```python
from build123d import *

# Parameters (mm, degrees)
SKETCH1_W            = 157.0786
SKETCH1_H            = 90.551
BOSS_EXTRUDE1_DEPTH  = 8
CUT_EXTRUDE21_DEPTH  = 5
FILLET8_R            = 2.75
SKETCH29_W           = 11.58993
SKETCH29_H           = 90.551
CUT_EXTRUDE25_DEPTH  = 182.486005463
FILLET9_R            = 5
SKETCH36_W           = 10
SKETCH36_H           = 10
SKETCH36_R           = 3.3
BOSS_EXTRUDE10_DEPTH = 8
FILLET10_R           = 2.5
CUT_EXTRUDE26_DEPTH  = 3


with BuildPart() as part:
    # Sketch1 → Boss-Extrude1 (new body)
    with BuildSketch(Plane(origin=(0, 0, 0), x_dir=(1, 0, 0), z_dir=(0, 1, 0))):
        with Locations((78.5393, -45.2755)):
            Rectangle(SKETCH1_W, SKETCH1_H)
    extrude(amount=BOSS_EXTRUDE1_DEPTH)

    # Sketch23 → Cut-Extrude21 (cut)
    with BuildSketch(Plane(origin=(0, 8, 0), x_dir=(1, 0, 0), z_dir=(0, 1, 0))):
        Polygon((140.6288, -86.4755), (23.2359173, -86.4755), (16.4498, -79.6893827), (16.4498, -10.8616173), (23.2359173, -4.0755), (140.6288, -4.0755), align=None)
    extrude(amount=-CUT_EXTRUDE21_DEPTH, mode=Mode.SUBTRACT)

    # Fillet8
    fillet8_edges = [part.edges().sort_by_distance(p)[0] for p in [
        (140.6288, 5.5, 4.0755),
        (140.6288, 5.5, 86.4755),
        (23.2359173, 5.5, 86.4755),
        (16.4498, 5.5, 79.6893827),
        (16.4498, 5.5, 10.8616173),
        (23.2359173, 5.5, 4.0755),
    ]]
    fillet(fillet8_edges, radius=FILLET8_R)

    # Sketch29 → Cut-Extrude25 (cut, through all)
    with BuildSketch(Plane(origin=(0, 8, 0), x_dir=(1, 0, 0), z_dir=(0, 1, 0))):
        with Locations((151.283635, -45.2755)):
            Rectangle(SKETCH29_W, SKETCH29_H)
        with Locations((5.794965, -45.2755)):
            Rectangle(SKETCH29_W, SKETCH29_H)
    extrude(amount=-CUT_EXTRUDE25_DEPTH, mode=Mode.SUBTRACT)

    # Fillet9
    fillet9_edges = [part.edges().sort_by_distance(p)[0] for p in [
        (145.48867, 4, 90.551),
        (145.48867, 4, 0),
        (11.58993, 4, 0),
        (11.58993, 4, 90.551),
    ]]
    fillet(fillet9_edges, radius=FILLET9_R)

    # Sketch36 → Boss-Extrude10 (add)
    # profile 1 of 4: a face of its own
    with BuildSketch(Plane.XZ):
        with Locations((25.6082, 95.551)):
            Rectangle(SKETCH36_W, SKETCH36_H)
        with Locations(Location((25.6082, 95.551, 0), (0, 0, 270))):
            Circle(SKETCH36_R, mode=Mode.SUBTRACT)
    # profile 2 of 4: a face of its own
    with BuildSketch(Plane.XZ):
        with Locations((128.3942697, 95.551)):
            Rectangle(SKETCH36_W, SKETCH36_H)
        with Locations(Location((128.3942697, 95.551, 0), (0, 0, 270))):
            Circle(SKETCH36_R, mode=Mode.SUBTRACT)
    # profile 3 of 4: a face of its own
    with BuildSketch(Plane.XZ):
        with Locations((25.6082, -5)):
            Rectangle(SKETCH36_W, SKETCH36_H)
        with Locations(Location((25.6082, -5, 0), (0, 0, 270))):
            Circle(SKETCH36_R, mode=Mode.SUBTRACT)
    # profile 4 of 4: a face of its own
    with BuildSketch(Plane.XZ):
        with Locations((128.3942697, -5)):
            Rectangle(SKETCH36_W, SKETCH36_H)
        with Locations(Location((128.3942697, -5, 0), (0, 0, 270))):
            Circle(SKETCH36_R, mode=Mode.SUBTRACT)
    extrude(amount=-BOSS_EXTRUDE10_DEPTH)

    # Fillet10
    fillet10_edges = [part.edges().sort_by_distance(p)[0] for p in [
        (20.6082, 4, 90.551),
        (20.6082, 4, 100.551),
        (30.6082, 4, 100.551),
        (30.6082, 4, 90.551),
        (123.3942697, 4, 90.551),
        (123.3942697, 4, 100.551),
        (133.3942697, 4, 100.551),
        (133.3942697, 4, 90.551),
        (30.6082, 4, 0),
        (30.6082, 4, -10),
        (20.6082, 4, -10),
        (20.6082, 4, 0),
        (123.3942697, 4, -10),
        (123.3942697, 4, 0),
        (133.3942697, 4, 0),
        (133.3942697, 4, -10),
    ]]
    fillet(fillet10_edges, radius=FILLET10_R)

    # Sketch37 → Cut-Extrude26 (cut)
    with BuildSketch(Plane(origin=(0, 3, 0), x_dir=(1, 0, 0), z_dir=(0, 1, 0))):
        Polygon((21.1393, -77.618314888), (24.996485112, -81.4755), (135.9393, -81.4755), (135.9393, -9.0755), (24.996485112, -9.0755), (21.1393, -12.932685112), align=None)
    extrude(amount=-CUT_EXTRUDE26_DEPTH, mode=Mode.SUBTRACT)


solid = part.part
```
Geometry check sheet. Reference: the model listing, model coordinates, mm. A direction names the side the tool comes from. Give positions to 0.01 mm unless a question says otherwise; leave off trailing zeros. Order: outer loops, then holes, each group sorted by start corner. A loop starts at its lowest first (then second) coordinate and runs counter-clockwise, first axis right, second up.
1. Gauge pin test, flat ends, axial feed: pin 1 Ø2 at (x, y) = (36, 6.5) entering from +Z; pin 2 Ø7.5 at (x, z) = (128.39, -5) entering from -Y; pin 3 Ø1.5 at (y, z) = (2, 95.5) entering from +X; pin 4 Ø1.5 at (x, y) = (124.5, 2.5) entering from +Z. Record the tip position at first contact, or that the pin passes through.
2. Access from +Z, -Z, +X, -X, +Y, -Y to the whole of each face (thin tool, end or side, straight path). Record for faces 4 (the face through (133.394, 4, 96)), 5 (the face through (123.394, 4, 96)), 6 (the face through (133.394, 4, -5)), 7 (the face through (20.608, 4, 96)).
3. Section check B-B, the plane z = -5. Enter the section's corners in (x, y), and give its area (3 significant figures).
4. Thickness scan on L1, parallel to X at y = 1.5, z = -5; L2, parallel to Z at x = 88.5, y = 4; L3, parallel to Z at x = 117.5, y = 1.75. Record the ranges inside material, lowest first.
5. Release check for a two-part mould opening along Z. For faces 1 (the face through (79, 3, 82)), 2 (the face through (30.608, 4, -5)), 3 (the face through (76, 4, 0)) record: pulls with the +Z half, pulls with the -Z half, needs draft (parallel to the pull), parting line crosses it, or undercut.
6. Section check A-A, the plane x = 73. Enter the section's corners in (y, z).
7. Section check D-D, the plane y = 1.5. Give the number of separate pieces and of enclosed holes in the cut face, and give its area (3 significant figures).
8. Section check C-C, the plane z = 15. Enter the section's corners in (x, y).
Values follow:
1. pin 1: stops at z = 90.55
1. pin 2: stops at y = 0
1. pin 3: stops at x = 133.39
1. pin 4: stops at z = 100.47
2. face 4: +Z, +X, +Y, -Y
2. face 5: +Z, +Y, -Y
2. face 6: -Z, +X, +Y, -Y
2. face 7: +Z, -X, +Y, -Y
3. outline: (20.61, 0) - (22.31, 0) - (22.31, 8) - (20.61, 8) - close; (28.91, 0) - (30.61, 0) - (30.61, 8) - (28.91, 8) - close; (123.39, 0) - (125.09, 0) - (125.09, 8) - (123.39, 8) - close; (131.69, 0) - (133.39, 0) - (133.39, 8) - (131.69, 8) - close
3. area: 54.4 mm2
4. L1: x = 20.61 to 22.31, 28.91 to 30.61, 123.39 to 125.09, 131.69 to 133.39
4. L2: z = 0 to 4.08, 86.48 to 90.55
4. L3: z = 0 to 9.08, 81.48 to 90.55
5. face 1: undercut
5. face 2: needs draft
5. face 3: pulls with the -Z half
6. outline: (0, 0) - (8, 0) - (8, 4.08) - (3, 4.08) - (3, 9.08) - (0, 9.08) - close; (0, 81.48) - (3, 81.48) - (3, 86.48) - (8, 86.48) - (8, 90.55) - (0, 90.55) - close
7. separate pieces: 1
7. enclosed holes: 5
7. area: 4,070 mm2
8. outline: (11.59, 0) - (21.14, 0) - (21.14, 3) - (16.45, 3) - (16.45, 8) - (11.59, 8) - close; (135.94, 0) - (145.49, 0) - (145.49, 8) - (140.63, 8) - (140.63, 3) - (135.94, 3) - close
